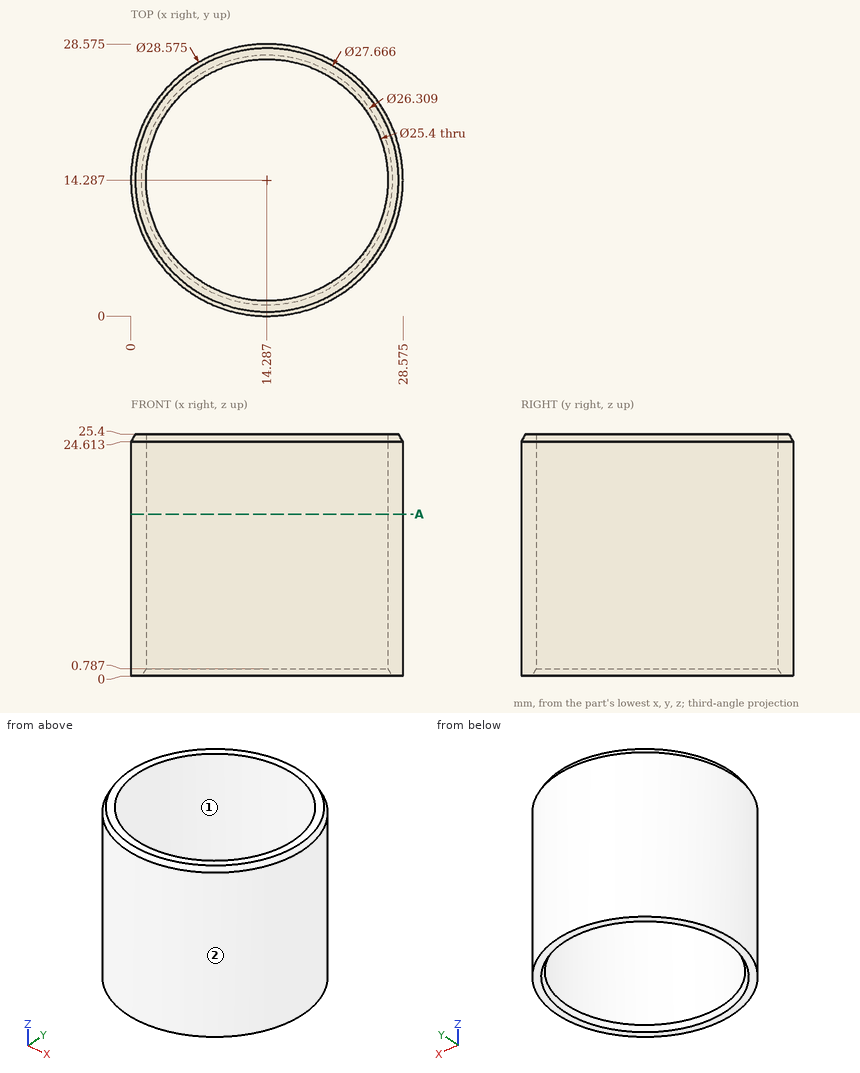
Geometry: see drawing. Coordinates: mm, zero at the bounding-box minimum. Round coordinates to 2 decimals unless told otherwise and drop trailing zeros. Write each loop counter-clockwise with the first axis right and the second up, starting at its lowest first coordinate (ties: lowest second). Pieces come first, ordered by that corner, then holes.
Item 1: Section query A-A (z = 17). Return loops of the section in (x, y) (1 decimal).
Item 2: Mould query, pull axis X, two halves, no side actions, for the marked faces 1 and 2. Classes: +X half, -X half, draft (parallel to the pull), parting line (faces both ways), or undercut.
Item 3: Pin query (flat end, axial travel): P1, Ø10, axis at x = 4.5, z = 19, coming from the -Y side (1 decimal); P2, Ø6, axis at x = 21.5, z = 13, coming from the +Y side; P3, Ø10, axis at x = 13, y = 8.5, coming from the +Z side; P4, Ø12, axis at y = 6.5, z = 11.5, coming from the -X side. Return the tip coordinate at first contact, or that it passes through.
Item 4: Material intervals for L1, parallel to Y at x = 16, z = 20.25; L2, parallel to X at y = 7.75, z = 7 (1 decimal); L3, parallel to X at y = 5.5, z = 7.5 (1 decimal), sorted ascending.
Completed:
1. outline: circle Ø28.6 at (14.3, 14.3); hole circle Ø25.4 at (14.3, 14.3)
2. face 1: undercut
2. face 2: parting line
3. P1: stops at y = 0.8
3. P2: stops at y = 27.94
3. P3: passes through
3. P4: stops at x = 0.11
4. L1: y = 0.1 to 1.7, 26.87 to 28.47
4. L2: x = 1.6 to 3.4, 25.2 to 27
4. L3: x = 3 to 5.1, 23.5 to 25.6
